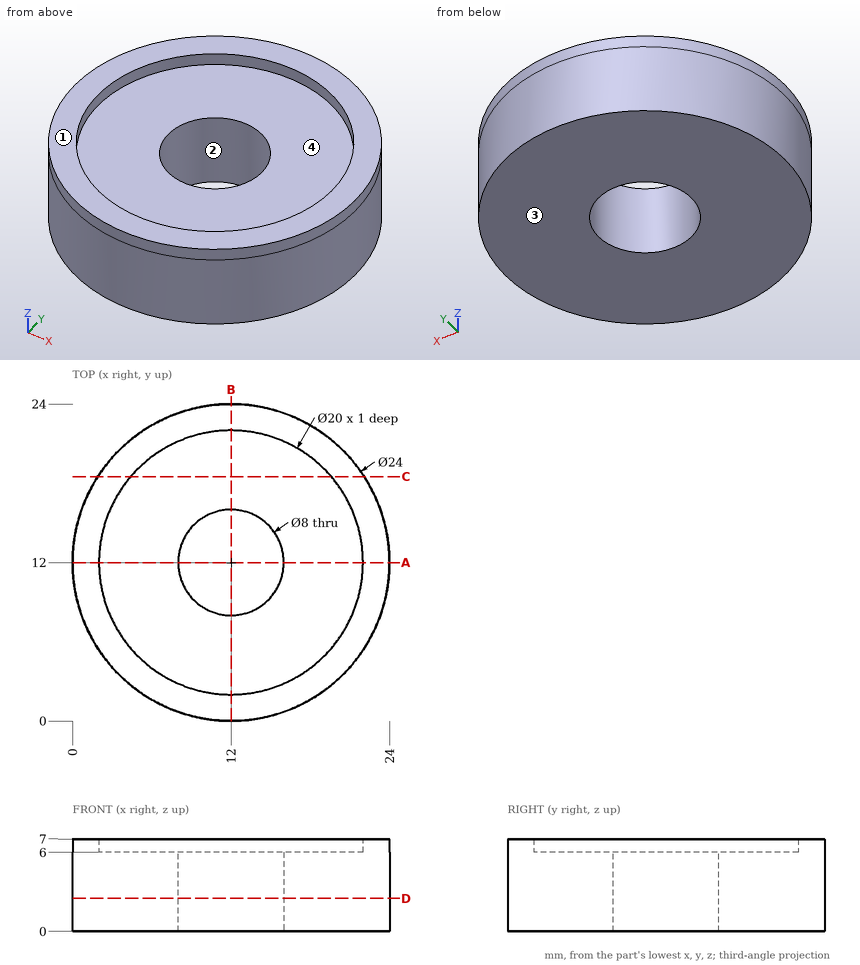
Geometry check sheet. Reference: drawing and pictorial views, mm from the part's lowest x, y, z. A direction names the side the tool comes from. Give positions to 0.01 mm unless a question says otherwise; leave off trailing zeros. Order: outer loops, then holes, each group sorted by start corner. A loop starts at its lowest first (then second) coordinate and runs counter-clockwise, first axis right, second up. Notation, with made-up numbers: M -8.75,57.5 L 35.25,57.5 A25 ccw 35.25,88.5 Z; hole C 17.5,15 d6. An arc over 180 degrees is marked long. Answer as a JSON object with one key per item and string values. Group by question number.
1) Mould release check, pull along Y, two halves, no side actions. Record for the marked faces 1 and 2: released by +Y, released by -Y, zero draft, split by the parting line, or undercut.
2) Scan lines: line 1 along Y through (x, z) = (12, 4.1); line 2 along Y through (x, z) = (12, 6.4); line 3 along Z through (x, y) = (18.75, 18). Record each from-to range of solid material in increasing order. Write a range as [from, to].
3) Access from +Z, -Z, +X, -X, +Y, -Y to the whole of each face (thin tool, end or side, straight path). Record for the marked faces 3 and 4.
4) Cross-section at C-C (y = 18.5). Enter the section's corners in (x, z), then the cut area to 3 significant figures.
5) Depth check by flat-ended pin: pin 1 Ø1 at (x, z) = (8, 3) entering from +Y; pin 2 Ø1 at (x, z) = (18, 2.5) entering from +Y; pin 3 Ø12 at (x, y) = (12, 12) entering from +Z. Enter the tip coordinate at first touch or a pass-through.
6) Cross-section at D-D (z = 2.5). Enter the section's corners in (x, y).
7) Cross-section at A-A (y = 12). Enter the section's corners in (x, z).
Result sheet:
{
 "1": {"face 1": "zero draft", "face 2": "undercut"},
 "2": {"line 1": "y = [0, 8], [16, 24]", "line 2": "y = [0, 2], [22, 24]", "line 3": "z = [0, 6]"},
 "3": {"face 3": "-Z, +X, -X, +Y, -Y", "face 4": "+Z"},
 "4": {"outline": "M 1.91,0 L 22.09,0 L 22.09,7 L 19.6,7 L 19.6,6 L 4.4,6 L 4.4,7 L 1.91,7 Z", "area": "126 mm2"},
 "5": {"pin 1": "stops at y = 23.48", "pin 2": "stops at y = 22.67", "pin 3": "stops at z = 6"},
 "6": {"outline": "C 12,12 d24; hole C 12,12 d8"},
 "7": {"outline": "M 0,0 L 8,0 L 8,6 L 2,6 L 2,7 L 0,7 Z; M 16,0 L 24,0 L 24,7 L 22,7 L 22,6 L 16,6 Z"}
}
